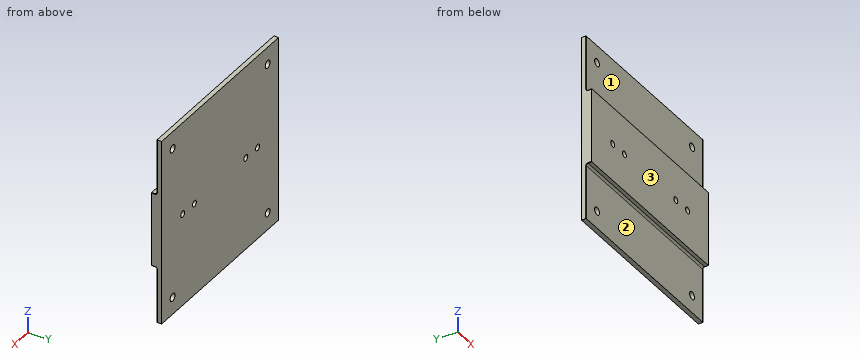
from build123d import *

# Parameters (mm, degrees)
SKETCH1_W           = 100
SKETCH1_H           = 100
SKETCH1_R           = 2.05
BOSS_EXTRUDE1_DEPTH = 2.5
SKETCH3_W           = 100
SKETCH3_H           = 40
BOSS_EXTRUDE2_DEPTH = 3
FILLET2_R           = 1
FILLET4_R           = 0.2
SKETCH4_R           = 1.65
CUT_EXTRUDE1_DEPTH  = 71.924255371


with BuildPart() as part:
    # Sketch1 → Boss-Extrude1 (new body)
    with BuildSketch(Plane(origin=(0, 0, 0), x_dir=(1, 0, 0), z_dir=(0, 1, 0))):
        Rectangle(SKETCH1_W, SKETCH1_H)
        with Locations(Location((-40.66, 40.66, 0), (0, 0, 270))):
            Circle(SKETCH1_R, mode=Mode.SUBTRACT)
        with Locations(Location((40.66, 40.66, 0), (0, 0, 270))):
            Circle(SKETCH1_R, mode=Mode.SUBTRACT)
        with Locations(Location((40.66, -40.66, 0), (0, 0, 270))):
            Circle(SKETCH1_R, mode=Mode.SUBTRACT)
        with Locations(Location((-40.66, -40.66, 0), (0, 0, 270))):
            Circle(SKETCH1_R, mode=Mode.SUBTRACT)
    extrude(amount=BOSS_EXTRUDE1_DEPTH)

    # Sketch3 → Boss-Extrude2 (add)
    with BuildSketch(Plane.XZ):
        Rectangle(SKETCH3_W, SKETCH3_H)
    extrude(amount=BOSS_EXTRUDE2_DEPTH)

    # Fillet2
    fillet2_edges = [part.edges().sort_by_distance(p)[0] for p in [
        (0, 0, 20),
        (0, 0, -20),
    ]]
    fillet(fillet2_edges, radius=FILLET2_R)

    # Fillet4
    fillet4_edges = [part.edges().sort_by_distance(p)[0] for p in [
        (50, -2, -20),
        (50, -2, 20),
        (-50, -2, 20),
        (-50, -2, -20),
        (50, 0, -35.5),
        (-50, 0, 35.5),
        (50, -0.292893219, -20.292893219),
        (-50, -0.292893219, -20.292893219),
        (-50, -0.292893219, 20.292893219),
        (50, -0.292893219, 20.292893219),
        (-50, 0, -35.5),
        (50, 0, 35.5),
    ]]
    fillet(fillet4_edges, radius=FILLET4_R)

    # Sketch4 → Cut-Extrude1 (cut, through all)
    with BuildSketch(Plane.XZ.offset(3)):
        with Locations(Location((-32, 0, 0), (0, 0, 270))):
            Circle(SKETCH4_R)
        with Locations(Location((-22, 0, 0), (0, 0, 270))):
            Circle(SKETCH4_R)
        with Locations(Location((22, 0, 0), (0, 0, 270))):
            Circle(SKETCH4_R)
        with Locations(Location((32, 0, 0), (0, 0, 270))):
            Circle(SKETCH4_R)
    extrude(amount=-CUT_EXTRUDE1_DEPTH, mode=Mode.SUBTRACT)


solid = part.part
The listing builds one solid part. Answer for the finished solid, in the listing's coordinates (mm). Face numbers are marked on the shaded views. A direction names the side the tool comes from. Round coordinates to 2 decimals unless told otherwise and drop trailing zeros. Write each loop counter-clockwise with the first axis right and the second up, starting at its lowest first coordinate (ties: lowest second). Pieces come first, ordered by that corner, then holes. Notation, with made-up numbers: M 65.25,55 L 120.25,55 A16 ccw 120.25,80 Z; hole C 85.25,-31 d4. An arc over 180 degrees is marked long. Write each question's results on one line, items separated by ' | '. Start each with the question number.
Item 1: Given pin 1 Ø1.6 at (x, y) = (-20, -2) entering from +Z; pin 2 Ø4.5 at (x, z) = (32, 0) entering from +Y; pin 3 Ø2 at (x, z) = (22, 0) entering from -Y; pin 4 Ø1 at (x, y) = (-9, -2.5) entering from -Z, each flat-ended and moving along its own axis, determine where each tip first touches the part or whether it passes through.
Item 2: Find section A-A on x = -40.66. Write down the section's boundary in (y, z), and give its area (3 significant figures).
Item 3: Straight lines are drawn through the part: probe 1 along X at (y, z) = (1.9, -40.66); probe 2 along X at (y, z) = (0.6, 0); probe 3 along X at (y, z) = (1.9, 40). For each, find the intervals that lie inside material, in ascending order.
Item 4: Find section B-B on y = -2.15. Write down the section's boundary in (x, z), and give its area (3 significant figures).
Item 5: Which of the six approach directions +Z, -Z, +X, -X, +Y, -Y give full straight-line access (tool end or side, diameter ignored) to the marked faces 1, 2 and 3?
Item 6: Find section D-D on z = 0. Write down the section's boundary in (x, y), and give its area (3 significant figures).
Item 7: Find section C-C on z = -40.66. Write down the section's boundary in (x, y), and give its area (3 significant figures).
Answer block:
1) pin 1: stops at z = 20 | pin 2: stops at y = 2.5 | pin 3: passes through | pin 4: stops at z = -20
2) outline: M -3,-20 L -1,-20 A1 cw 0,-21 L 0,-38.61 L 2.5,-38.61 L 2.5,38.61 L 0,38.61 L 0,21 A1 cw -1,20 L -3,20 Z; M 0,-50 L 2.5,-50 L 2.5,-42.71 L 0,-42.71 Z; M 0,42.71 L 2.5,42.71 L 2.5,50 L 0,50 Z | area: 350 mm²
3) probe 1: x = -50 to -42.71, -38.61 to 38.61, 42.71 to 50 | probe 2: x = -50 to -33.65, -30.35 to -23.65, -20.35 to 20.35, 23.65 to 30.35, 33.65 to 50 | probe 3: x = -50 to -42.6, -38.72 to 38.72, 42.6 to 50
4) outline: M -50,-19.8 A0.2 ccw -49.8,-20 L 49.8,-20 A0.2 ccw 50,-19.8 L 50,19.8 A0.2 ccw 49.8,20 L -49.8,20 A0.2 ccw -50,19.8 Z; hole C -32,0 d3.3; hole C -22,0 d3.3; hole C 22,0 d3.3; hole C 32,0 d3.3 | area: 3,970 mm²
5) face 1: +Z, +X, -X, -Y | face 2: -Z, +X, -X, -Y | face 3: +Z, -Z, +X, -X, -Y
6) outline: M -50,-3 L -33.65,-3 L -33.65,2.5 L -50,2.5 Z; M -30.35,-3 L -23.65,-3 L -23.65,2.5 L -30.35,2.5 Z; M -20.35,-3 L 20.35,-3 L 20.35,2.5 L -20.35,2.5 Z; M 23.65,-3 L 30.35,-3 L 30.35,2.5 L 23.65,2.5 Z; M 33.65,-3 L 50,-3 L 50,2.5 L 33.65,2.5 Z | area: 477 mm²
7) outline: M -50,0.2 A0.2 ccw -49.8,0 L -42.71,0 L -42.71,2.5 L -50,2.5 Z; M -38.61,0 L 38.61,0 L 38.61,2.5 L -38.61,2.5 Z; M 42.71,0 L 49.8,0 A0.2 ccw 50,0.2 L 50,2.5 L 42.71,2.5 Z | area: 229 mm²
